from build123d import *

# Parameters (mm, degrees)
SKETCH1_R           = 1.6
BOSS_EXTRUDE1_DEPTH = 3


with BuildPart() as part:
    # Sketch1 → Boss-Extrude1 (new body)
    with BuildSketch(Plane(origin=(0, 0, 0), x_dir=(1, 0, 0), z_dir=(0, 1, 0))):
        with BuildLine():
            Line((-70, 42.5), (70, 42.5))
            ThreePointArc((70, 42.5), (73.535533906, 41.035533906), (75, 37.5))
            Line((75, 37.5), (75, -37.5))
            ThreePointArc((75, -37.5), (73.535533906, -41.035533906), (70, -42.5))
            Line((70, -42.5), (-70, -42.5))
            ThreePointArc((-70, -42.5), (-73.535533906, -41.035533906), (-75, -37.5))
            Line((-75, -37.5), (-75, 37.5))
            ThreePointArc((-75, 37.5), (-73.535533906, 41.035533906), (-70, 42.5))
        make_face()
        with Locations(Location((-65, 8, 0), (0, 0, 270))):
            Circle(SKETCH1_R, mode=Mode.SUBTRACT)
        with Locations(Location((-65, -8, 0), (0, 0, 90))):
            Circle(SKETCH1_R, mode=Mode.SUBTRACT)
        with Locations(Location((-51, 8, 0), (0, 0, 90))):
            Circle(SKETCH1_R, mode=Mode.SUBTRACT)
        with Locations(Location((-51, -8, 0), (0, 0, 270))):
            Circle(SKETCH1_R, mode=Mode.SUBTRACT)
        with Locations(Location((51, -8, 0), (0, 0, 90))):
            Circle(SKETCH1_R, mode=Mode.SUBTRACT)
        with Locations(Location((51, 8, 0), (0, 0, 270))):
            Circle(SKETCH1_R, mode=Mode.SUBTRACT)
        with Locations(Location((65, -8, 0), (0, 0, 270))):
            Circle(SKETCH1_R, mode=Mode.SUBTRACT)
        with Locations(Location((65, 8, 0), (0, 0, 90))):
            Circle(SKETCH1_R, mode=Mode.SUBTRACT)
        with Locations(Location((-27.81, 19.29, 0), (0, 0, 270))):
            Circle(SKETCH1_R, mode=Mode.SUBTRACT)
        with Locations(Location((-27.81, 0, 0), (0, 0, 270))):
            Circle(SKETCH1_R, mode=Mode.SUBTRACT)
        with Locations(Location((-27.81, -19.29, 0), (0, 0, 90))):
            Circle(SKETCH1_R, mode=Mode.SUBTRACT)
        with Locations(Location((27.81, -19.29, 0), (0, 0, 270))):
            Circle(SKETCH1_R, mode=Mode.SUBTRACT)
        with Locations(Location((27.81, 19.29, 0), (0, 0, 90))):
            Circle(SKETCH1_R, mode=Mode.SUBTRACT)
        with Locations(Location((27.81, 0, 0), (0, 0, 90))):
            Circle(SKETCH1_R, mode=Mode.SUBTRACT)
        with Locations(Location((-70, 37.5, 0), (0, 0, 270))):
            Circle(SKETCH1_R, mode=Mode.SUBTRACT)
        with Locations(Location((-70, -37.5, 0), (0, 0, 90))):
            Circle(SKETCH1_R, mode=Mode.SUBTRACT)
        with Locations(Location((70, -37.5, 0), (0, 0, 270))):
            Circle(SKETCH1_R, mode=Mode.SUBTRACT)
        with Locations(Location((70, 37.5, 0), (0, 0, 90))):
            Circle(SKETCH1_R, mode=Mode.SUBTRACT)
        with BuildLine():
            Line((28, 32.5), (28, 36.5))
            ThreePointArc((28, 36.5), (27.414213562, 37.914213562), (26, 38.5))
            Line((26, 38.5), (-26, 38.5))
            ThreePointArc((-26, 38.5), (-27.414213562, 37.914213562), (-28, 36.5))
            Line((-28, 36.5), (-28, 32.5))
            ThreePointArc((-28, 32.5), (-27.414213562, 31.085786438), (-26, 30.5))
            Line((-26, 30.5), (26, 30.5))
            ThreePointArc((26, 30.5), (27.414213562, 31.085786438), (28, 32.5))
        make_face(mode=Mode.SUBTRACT)
        with BuildLine():
            Line((-26, -30.5), (26, -30.5))
            ThreePointArc((26, -30.5), (27.414213562, -31.085786438), (28, -32.5))
            Line((28, -32.5), (28, -36.5))
            ThreePointArc((28, -36.5), (27.414213562, -37.914213562), (26, -38.5))
            Line((26, -38.5), (-26, -38.5))
            ThreePointArc((-26, -38.5), (-27.414213562, -37.914213562), (-28, -36.5))
            Line((-28, -36.5), (-28, -32.5))
            ThreePointArc((-28, -32.5), (-27.414213562, -31.085786438), (-26, -30.5))
        make_face(mode=Mode.SUBTRACT)
        with BuildLine():
            Line((-38.81, 32.5), (-38.81, 36.5))
            ThreePointArc((-38.81, 36.5), (-39.395786438, 37.914213562), (-40.81, 38.5))
            Line((-40.81, 38.5), (-60.81, 38.5))
            ThreePointArc((-60.81, 38.5), (-62.224213562, 37.914213562), (-62.81, 36.5))
            Line((-62.81, 36.5), (-62.81, 32.5))
            ThreePointArc((-62.81, 32.5), (-62.224213562, 31.085786438), (-60.81, 30.5))
            Line((-60.81, 30.5), (-40.81, 30.5))
            ThreePointArc((-40.81, 30.5), (-39.395786438, 31.085786438), (-38.81, 32.5))
        make_face(mode=Mode.SUBTRACT)
        with BuildLine():
            Line((-60.81, -30.5), (-40.81, -30.5))
            ThreePointArc((-40.81, -30.5), (-39.395786438, -31.085786438), (-38.81, -32.5))
            Line((-38.81, -32.5), (-38.81, -36.5))
            ThreePointArc((-38.81, -36.5), (-39.395786438, -37.914213562), (-40.81, -38.5))
            Line((-40.81, -38.5), (-60.81, -38.5))
            ThreePointArc((-60.81, -38.5), (-62.224213562, -37.914213562), (-62.81, -36.5))
            Line((-62.81, -36.5), (-62.81, -32.5))
            ThreePointArc((-62.81, -32.5), (-62.224213562, -31.085786438), (-60.81, -30.5))
        make_face(mode=Mode.SUBTRACT)
        with BuildLine():
            Line((38.81, 32.5), (38.81, 36.5))
            ThreePointArc((38.81, 36.5), (39.395786438, 37.914213562), (40.81, 38.5))
            Line((40.81, 38.5), (60.81, 38.5))
            ThreePointArc((60.81, 38.5), (62.224213562, 37.914213562), (62.81, 36.5))
            Line((62.81, 36.5), (62.81, 32.5))
            ThreePointArc((62.81, 32.5), (62.224213562, 31.085786438), (60.81, 30.5))
            Line((60.81, 30.5), (40.81, 30.5))
            ThreePointArc((40.81, 30.5), (39.395786438, 31.085786438), (38.81, 32.5))
        make_face(mode=Mode.SUBTRACT)
        with BuildLine():
            Line((38.81, -32.5), (38.81, -36.5))
            ThreePointArc((38.81, -36.5), (39.395786438, -37.914213562), (40.81, -38.5))
            Line((40.81, -38.5), (60.81, -38.5))
            ThreePointArc((60.81, -38.5), (62.224213562, -37.914213562), (62.81, -36.5))
            Line((62.81, -36.5), (62.81, -32.5))
            ThreePointArc((62.81, -32.5), (62.224213562, -31.085786438), (60.81, -30.5))
            Line((60.81, -30.5), (40.81, -30.5))
            ThreePointArc((40.81, -30.5), (39.395786438, -31.085786438), (38.81, -32.5))
        make_face(mode=Mode.SUBTRACT)
    extrude(amount=BOSS_EXTRUDE1_DEPTH)


solid = part.part
Could you check a few things on this model? Use its own coordinates, in mm. A direction names the side the tool comes from. Coordinates: 2 decimals unless noted, no trailing zeros. Order: outer loops, then holes, each group sorted by start corner. A loop starts at its lowest first (then second) coordinate and runs counter-clockwise, first axis right, second up. Notation, with made-up numbers: (56.25, 40.25) -> (72.25, 40.25) arc R28 ccw to (72.25, 59.25) -> close; hole circle Ø4 at (-18.5, -6.5). An arc over 180 degrees is marked (long way). One line per item, written item: value. Start each with the question number.
1) Imagine slicing it at A-A on x = -43.5. List the corners of the cut face in (y, z) for me.
2) If I drill on L1, parallel to X at y = 1.2, z = 19.29; L2, parallel to X at y = 1.2, z = 35; L3, parallel to Z at x = 21, y = 1.5, over which ranges is the centre line in solid material (lowest first)? Write a range as [from, to].
3) Which directions (+Z, -Z, +X, -X, +Y, -Y) give clear straight access to the entire face, cutting with the end or side of a thin tool? Please do faces 1 (the cylindrical face through (-73.57, 1.48, -41)), 2 (the flat face through (-51, 1, -38.5)).
4) Imagine slicing it at C-C on y = 1.3. Count the separate pieces of the cut face and the enclosed holes in it, plus the area to 3 significant figures.
5) Imagine slicing it at B-B on z = 0. List the corners of the cut face in (x, y) for me, plus the area to 3 significant figures.
6) We'd pull the mould along X, two halves only. Please class faces 3 (the cylindrical face through (29.4, 1.5, 19.1)), 4 (the flat face through (1, 0, -1)), 5 (the flat face through (75, 1, -1)): +X half, -X half, draft (parallel to the pull), parting line (faces both ways), or undercut.
Answer list:
1. outline: (0, -42.5) -> (3, -42.5) -> (3, -38.5) -> (0, -38.5) -> close; (0, -30.5) -> (3, -30.5) -> (3, 30.5) -> (0, 30.5) -> close; (0, 38.5) -> (3, 38.5) -> (3, 42.5) -> (0, 42.5) -> close
2. L1: x = [-75, -29.41], [-26.21, 26.21], [29.41, 75]
2. L2: x = [-75, -62.81], [-38.81, -28], [28, 38.81], [62.81, 75]
2. L3: z = [-42.5, -38.5], [-30.5, 30.5], [38.5, 42.5]
3. face 1: -Z, -X, +Y, -Y
3. face 2: +Y, -Y
4. separate pieces: 1
4. enclosed holes: 24
4. area: 10,900 mm2
5. outline: (-75, 0) -> (-29.41, 0) -> (-29.41, 3) -> (-75, 3) -> close; (-26.21, 0) -> (26.21, 0) -> (26.21, 3) -> (-26.21, 3) -> close; (29.41, 0) -> (75, 0) -> (75, 3) -> (29.41, 3) -> close
5. area: 431 mm2
6. face 3: undercut
6. face 4: draft
6. face 5: +X half
